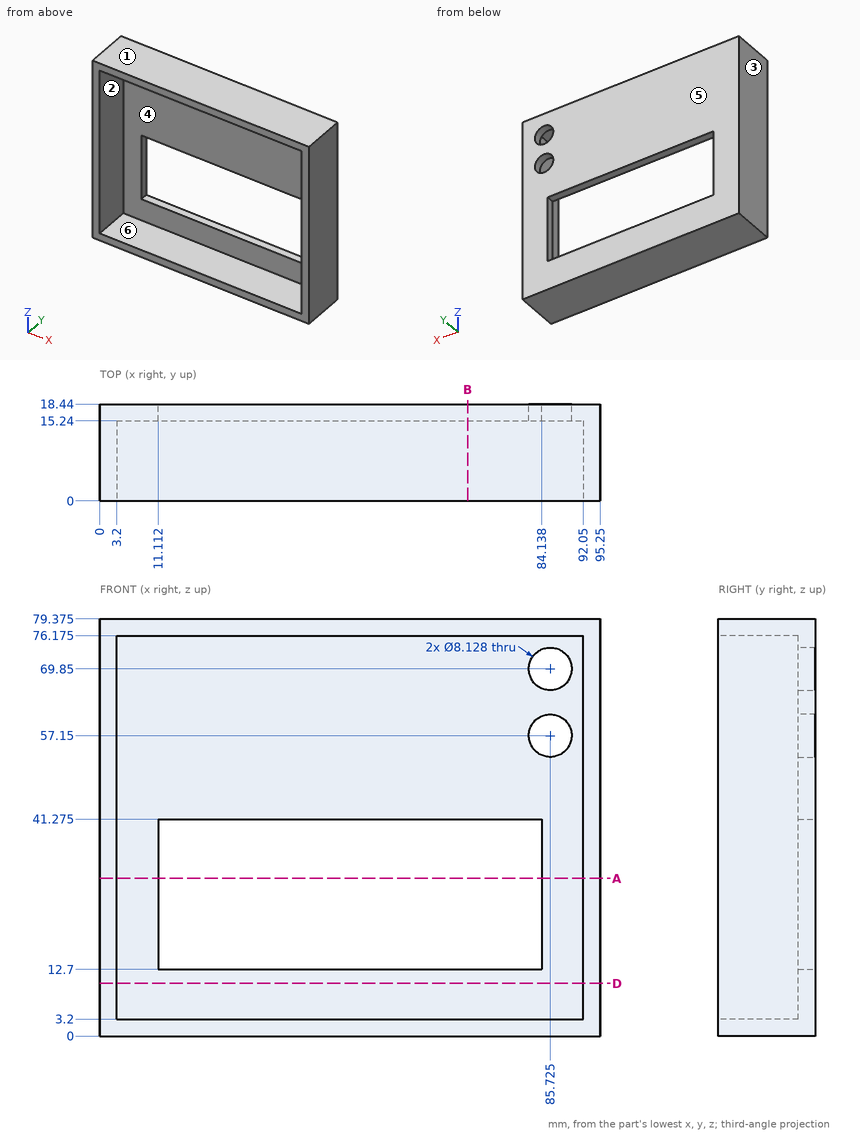
Job drawing, mm, ordinate dimensions from the low corner. One solid piece. A direction names the side the tool comes from. Round coordinates to 2 decimals unless told otherwise and drop trailing zeros. Loops run counter-clockwise (first coordinate to the right, second up) from the corner with the lowest first, then second, coordinate; pieces in that order, holes last. Notation, with made-up numbers: M -37.5,0 L -5.5,0 A27 ccw -5.5,22 Z; hole C 31,22.5 d8. An arc over 180 degrees is marked long. One line per question, with ' | ' between items. Start each with the question number.
Item 1: Cut at A-A, the plane z = 30. Write the cut outline in (x, y), plus the area to 3 significant figures.
Item 2: Two-plate mould, pull along X, no slides. Class the marked faces 1, 2, 3 and 4: pulls with the +X half, pulls with the -X half, needs draft (parallel to the pull), parting line crosses it, or undercut.
Item 3: Wall check: line 1 (X direction, y = 15.9, z = 69.85); line 2 (Z direction, x = 69, y = 13.25) (1 decimal); line 3 (X direction, y = 6.5, z = 18). Give the ranges that are in metal, low to high.
Item 4: Which spindle directions (+Z, -Z, +X, -X, +Y, -Y) get a long thin tool onto all of the face, cutting with end or side? Do the marked faces 5 and 6. Say none if no direction does.
Item 5: Cut at B-B, the plane x = 70. Write the cut outline in (y, z) (1 decimal).
Item 6: Pin check, flat tip, straight feed: pin 1 Ø12 at (x, z) = (15.5, 67) entering from -Y. Stop position of the tip, or through.
Item 7: Cut at D-D, the plane z = 10. Write the cut outline in (x, y).
Responses:
1) outline: M 0,0 L 3.2,0 L 3.2,15.24 L 11.11,15.24 L 11.11,18.44 L 0,18.44 Z; M 84.14,15.24 L 92.05,15.24 L 92.05,0 L 95.25,0 L 95.25,18.44 L 84.14,18.44 Z | area: 169 mm²
2) face 1: needs draft | face 2: undercut | face 3: pulls with the -X half | face 4: undercut
3) line 1: x = 0 to 81.66, 89.79 to 95.25 | line 2: z = 0 to 3.2, 76.2 to 79.4 | line 3: x = 0 to 3.2, 92.05 to 95.25
4) face 5: +Z, -Z, +X, -X, +Y | face 6: -Y
5) outline: M 0,0 L 18.4,0 L 18.4,12.7 L 15.2,12.7 L 15.2,3.2 L 0,3.2 Z; M 0,76.2 L 15.2,76.2 L 15.2,41.3 L 18.4,41.3 L 18.4,79.4 L 0,79.4 Z
6) pin 1: stops at y = 15.24
7) outline: M 0,0 L 3.2,0 L 3.2,15.24 L 92.05,15.24 L 92.05,0 L 95.25,0 L 95.25,18.44 L 0,18.44 Z
